Part model, mm, in its own coordinate system. Coordinates: 2 decimals unless noted, no trailing zeros. Write each loop counter-clockwise with the first axis right and the second up, starting at its lowest first coordinate (ties: lowest second). Pieces come first, ordered by that corner, then holes. Notation, with made-up numbers: (43.5, 44.5) - (62.5, 44.5) arc R19 ccw to (62.5, 49.5) - close; hole circle Ø5 at (22.5, 72.5). An arc over 180 degrees is marked (long way). Use a Markdown table: item, result.
```python
from build123d import *

# Parameters (mm, degrees)
THICKEN1_T1          = 0.625
M2_CLEARANCE_HOLE1_D = 2.4


with BuildPart() as body_1:
    # Sketch1 → Surface-Fill1: a flat surface bounded by the sketch
    with BuildSketch(Plane(origin=(0, 0, 0), x_dir=(1, 0, 0), z_dir=(0, 1, 0)), mode=Mode.PRIVATE) as surface_fill1_1_region:
        with BuildLine():
            Line((-25.4, -75.628621566), (25.4, -75.628621566))
            ThreePointArc((25.4, -75.628621566), (0, 79.78), (-25.4, -75.628621566))
        make_face()
        with BuildLine():
            Line((-25.4, -71.396417277), (25.4, -71.396417277))
            ThreePointArc((25.4, -71.396417277), (0, 75.78), (-25.4, -71.396417277))
        make_face(mode=Mode.SUBTRACT)
    surface_fill1_1 = surface_fill1_1_region.sketch.faces()[0]
    add(Solid.thicken(surface_fill1_1, THICKEN1_T1))

    # M2 Clearance Hole1 (through all)
    with Locations(Plane(origin=(0, 0.625, 0), x_dir=(1, 0, 0), z_dir=(0, 1, 0))):
        with Locations((0, 77.529954233), (0, -73.744874158), (77.744469628, -0.179745534), (-77.678576515, -0.083327834), (56.371935899, 53.45957237), (-59.482060021, 50.023142165), (61.035706748, -48.220860015), (-60.982517002, -48.258309848)):
            Hole(M2_CLEARANCE_HOLE1_D / 2)


solid = body_1.part
```
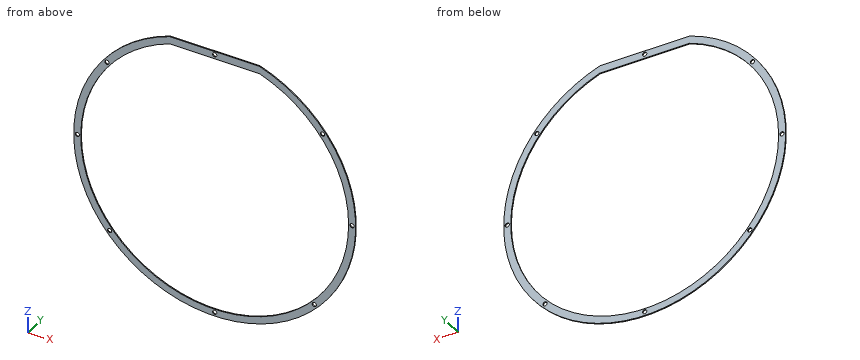
Item 1: Band-saw the part on A-A, the plane z = -9. Give the cut face in (x, y) (3 decimals), then the cut area to 3 significant figures.
From the geometry:
| item | result |
|---|---|
| outline | (-79.271, 0) - (-75.244, 0) - (-75.244, 0.625) - (-79.271, 0.625) - close; (75.244, 0) - (79.271, 0) - (79.271, 0.625) - (75.244, 0.625) - close |
| area | 5.03 mm^2 |
Item 2: Drill centre lines: probe 1 along Z at (x, y) = (0, 0.55); probe 2 along X at (y, z) = (0.25, 0); probe 3 along X at (y, z) = (0.4, 6). Where is each one in solid material? Low to high.
From the geometry:
| item | result |
|---|---|
| probe 1 | -79.78 to -78.73, -76.33 to -75.78, 71.4 to 72.54, 74.94 to 75.63 |
| probe 2 | -79.78 to -78.88, -76.48 to -75.78, 75.78 to 76.56, 78.93 to 79.78 |
| probe 3 | -79.55 to -75.54, 75.54 to 79.55 |
Item 3: Band-saw the part on B-B, the plane x = -38. Give the cut face in (y, z) (3 decimals), then the cut area to 3 significant figures.
From the geometry:
| item | result |
|---|---|
| outline | (0, -70.149) - (0.625, -70.149) - (0.625, -65.564) - (0, -65.564) - close; (0, 65.564) - (0.625, 65.564) - (0.625, 70.149) - (0, 70.149) - close |
| area | 5.73 mm^2 |
Item 4: Drop a flat-ended pin along its axis: P1, Ø1.4, axis at x = 61.04, z = 48.22, coming from the -Y side. Give the stop position or say it passes through.
From the geometry:
| item | result |
|---|---|
| P1 | through |
Item 5: Band-saw the part on C-C, the plane y = 0.45. Count the separate pieces of the cut face and the enclosed holes in it, then the cut area to 3 significant figures.
From the geometry:
| item | result |
|---|---|
| separate pieces | 1 |
| enclosed holes | 9 |
| area | 1,930 mm^2 |
